Check sheet for the drawn part. Datum: minimum x, y, z corner. Units: mm. Coordinates: 2 decimals unless noted, no trailing zeros. Loops run counter-clockwise (first coordinate to the right, second up) from the corner with the lowest first, then second, coordinate; pieces in that order, holes last.
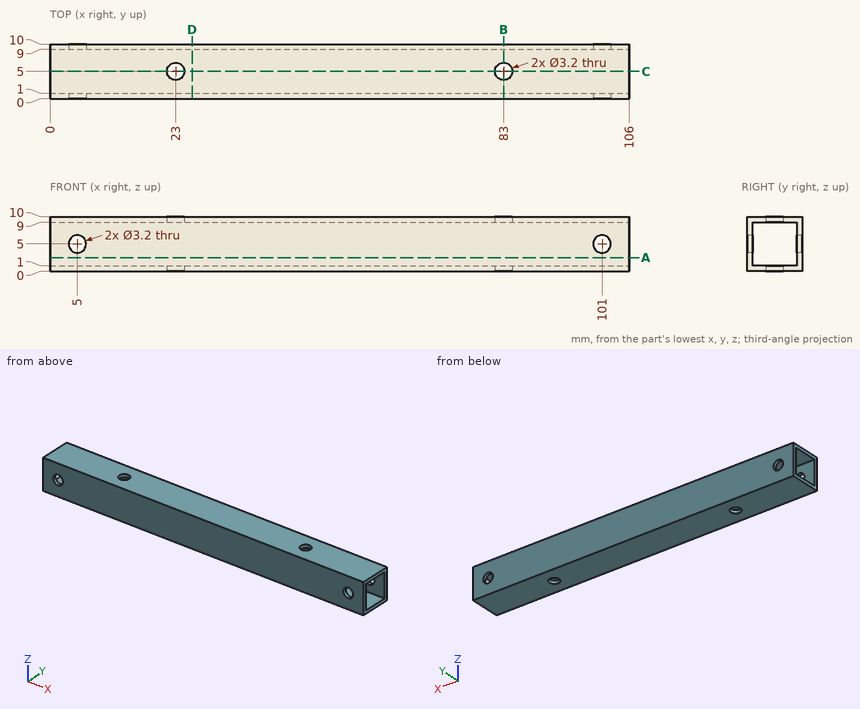
(1) Sectioned sample at B-B on x = 83. Record the cut outline in (y, z).
Findings:
outline: (0, 0) - (3.4, 0) - (3.4, 1) - (1, 1) - (1, 9) - (3.4, 9) - (3.4, 10) - (0, 10) - close; (6.6, 0) - (10, 0) - (10, 10) - (6.6, 10) - (6.6, 9) - (9, 9) - (9, 1) - (6.6, 1) - close
(2) Gauge pin test, flat end, axial feed: pin 1 Ø2.5 at (x, z) = (5, 5) entering from -Y. Record the tip position at first contact, or that the pin passes through.
Findings:
pin 1: passes through
(3) Sectioned sample at C-C on y = 5. Record the cut outline in (x, z).
Findings:
outline: (0, 0) - (21.4, 0) - (21.4, 1) - (0, 1) - close; (0, 9) - (21.4, 9) - (21.4, 10) - (0, 10) - close; (24.6, 0) - (81.4, 0) - (81.4, 1) - (24.6, 1) - close; (24.6, 9) - (81.4, 9) - (81.4, 10) - (24.6, 10) - close; (84.6, 0) - (106, 0) - (106, 1) - (84.6, 1) - close; (84.6, 9) - (106, 9) - (106, 10) - (84.6, 10) - close
(4) Scan lines: L1, parallel to X at y = 9.75, z = 5; L2, parallel to Z at x = 21, y = 5. Record each from-to range of solid material in increasing order.
Findings:
L1: x = 0 to 3.4, 6.6 to 99.4, 102.6 to 106
L2: z = 0 to 1, 9 to 10
(5) Sectioned sample at D-D on x = 26. Record the cut outline in (y, z).
Findings:
outline: (0, 0) - (10, 0) - (10, 10) - (0, 10) - close; hole (1, 1) - (9, 1) - (9, 9) - (1, 9) - close
(6) Sectioned sample at A-A on z = 2.5. Record the cut outline in (x, y), and give its area (3 significant figures).
Findings:
outline: (0, 0) - (106, 0) - (106, 1) - (0, 1) - close; (0, 9) - (106, 9) - (106, 10) - (0, 10) - close
area: 212 mm2
